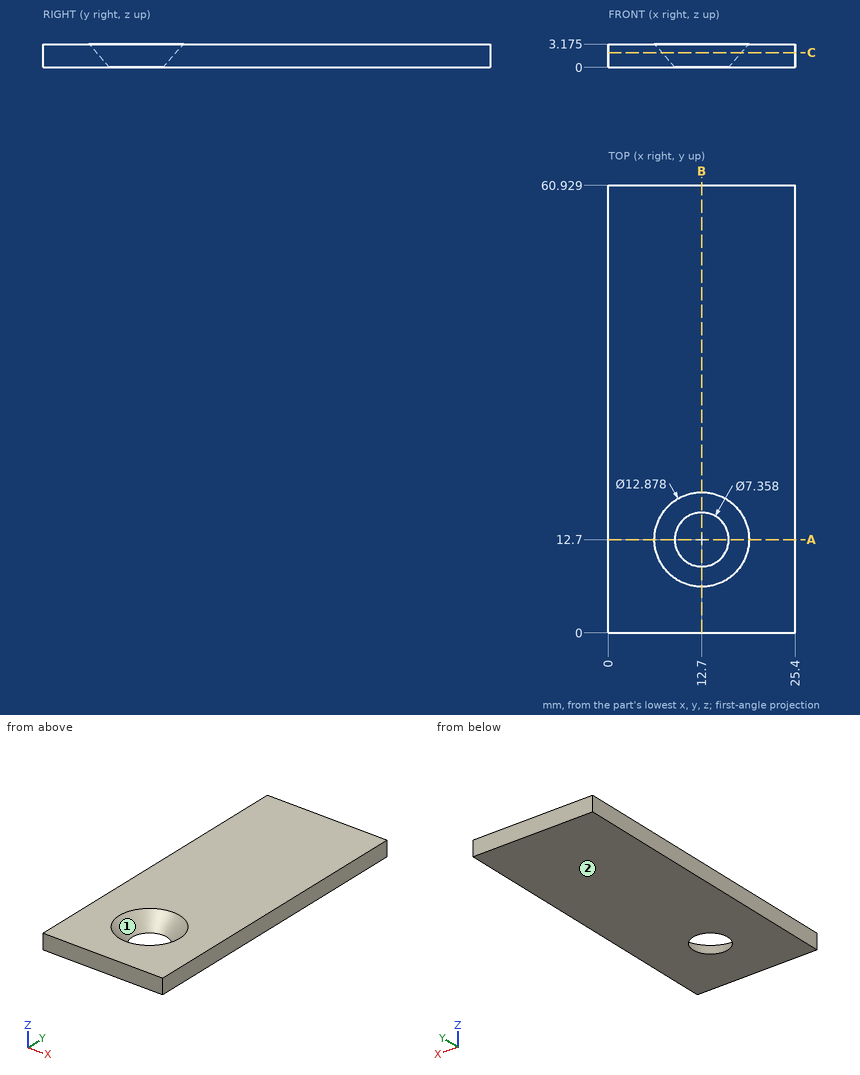
The drawing under review shows one solid part. Ordinate dimensions are in mm from its lowest x, y, z. Give positions to 0.01 mm unless a question says otherwise; leave off trailing zeros. Write each loop counter-clockwise with the first axis right and the second up, starting at its lowest first coordinate (ties: lowest second). Pieces come first, ordered by that corner, then holes. Notation, with made-up numbers: (78, 9) - (122, 9) arc R29 cw to (122, 41) - close; hole circle Ø5 at (4, 64.25). An arc over 180 degrees is marked (long way). Answer in a Markdown table with one row per item. Add a question column.
1. We need section A-A on y = 12.7. Write out the cut boundary in (x, z) (1 decimal).
2. We need section C-C on z = 2. Write out the cut boundary in (x, y) (1 decimal), then the cut area to 3 significant figures.
3. Wall thickness on line 1 along Y through (x, z) = (13.5, 1.25); line 2 along Y through (x, z) = (10.5, 1.85); line 3 along X through (y, z) = (15.5, 1.35): over which ranges is each line inside the solid? List them lowest first. Write a range as [from, to].
4. Draft analysis for pull direction Y (two halves, no side actions). For the marked faces 1 and 2, state which applies: +Y half, -Y half, draft (parallel to the pull), parting line (faces both ways), or undercut.
5. Insertion check: P1, Ø1, axis at y = 44, z = 1, coming from the -X side. The pin has a flat end and moves straight along its axis. Give the tip position at first contact, or say it passes through.
6. We need section B-B on x = 12.7. Write out the cut boundary in (y, z) (1 decimal).
Ans:
| question | item | result |
|---|---|---|
| 1 | outline | (0, 0) - (9, 0) - (6.3, 3.2) - (0, 3.2) - close; (16.4, 0) - (25.4, 0) - (25.4, 3.2) - (19.1, 3.2) - close |
| 2 | outline | (0, 0) - (25.4, 0) - (25.4, 60.9) - (0, 60.9) - close; hole circle Ø10.8 at (12.7, 12.7) |
| 2 | area | 1,460 mm^2 |
| 3 | line 1 | y = [0, 8], [17.4, 60.93] |
| 3 | line 2 | y = [0, 7.89], [17.51, 60.93] |
| 3 | line 3 | x = [0, 8.74], [16.66, 25.4] |
| 4 | face 1 | undercut |
| 4 | face 2 | draft |
| 5 | P1 | stops at x = 0 |
| 6 | outline | (0, 0) - (9, 0) - (6.3, 3.2) - (0, 3.2) - close; (16.4, 0) - (60.9, 0) - (60.9, 3.2) - (19.1, 3.2) - close |
